Here's how the part is built. I have some questions about the finished solid (model axes, mm). Face numbers are marked on the shaded views. A direction names the side the tool comes from. Give positions to 0.01 mm unless a question says otherwise; leave off trailing zeros. Loops run counter-clockwise (first coordinate to the right, second up) from the corner with the lowest first, then second, coordinate; pieces in that order, holes last. Notation, with made-up numbers: (-11.75, 37) - (29.25, 37) arc R9 cw to (29.25, 50) - close; hole circle Ø6 at (54.5, 31). An arc over 180 degrees is marked (long way). One line per item, written item: value. Start each with the question number.
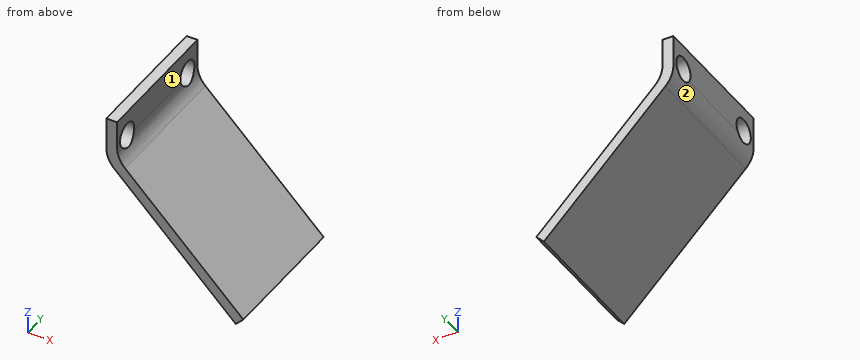
```python
from build123d import *

# Parameters (mm, degrees)
SKETCH1_W               = 1
SKETCH1_H               = 4
BOSS_EXTRUDE1_DEPTH     = 12.7
BOSS_EXTRUDE2_DEPTH     = 12.7
FILLET1_R               = 2.54
SKETCH3_R               = 1.125
CUT_EXTRUDE1_DEPTH      = 24.536198366
CUT_EXTRUDE1_DEPTH_BACK = 24.536198366


with BuildPart() as part:
    # Sketch1 → Boss-Extrude1 (new body)
    with BuildSketch(Plane(origin=(0, 0, 0), x_dir=(1, 0, 0), z_dir=(0, 1, 0))):
        with Locations((0.5, 2)):
            Rectangle(SKETCH1_W, SKETCH1_H)
    extrude(amount=BOSS_EXTRUDE1_DEPTH)

    # Sketch2 → Boss-Extrude2 (add)
    with BuildSketch(Plane(origin=(0, 0, 0), x_dir=(1, 0, 0), z_dir=(0, 1, 0))):
        Polygon((0, 4), (11.992893219, 15.992893219), (12.7, 15.285786438), (0.707106781, 3.292893219), align=None)
    extrude(amount=BOSS_EXTRUDE2_DEPTH)

    # Fillet1
    fillet1_edges = [part.edges().sort_by_distance(p)[0] for p in [
        (1, 6.35, -3.585786438),
        (0, 6.35, -4),
    ]]
    fillet(fillet1_edges, radius=FILLET1_R)

    # Sketch3 → Cut-Extrude1 (cut, two sides)
    with BuildSketch(Plane(origin=(1, 0, 0), x_dir=(0, 0, -1), z_dir=(1, 0, 0))) as cut_extrude1_sk:
        with Locations(Location((2.276792488, 11.1125, 0), (0, 0, 306.622338606))):
            Circle(SKETCH3_R)
        with Locations(Location((2.276792488, 1.5875, 0), (0, 0, 306.622338606))):
            Circle(SKETCH3_R)
    extrude(amount=CUT_EXTRUDE1_DEPTH, mode=Mode.SUBTRACT)
    extrude(cut_extrude1_sk.sketch, amount=-CUT_EXTRUDE1_DEPTH_BACK, mode=Mode.SUBTRACT)


solid = part.part
```
(1) If we section it at D-D on x = 3.5: List the corners of the cut face in (y, z) for me.
(2) If we section it at B-B on y = 6.5: List the corners of the cut face in (x, z) for me.
(3) Will these pins go through, and if not, where does the flat tip stop? pin 1 (1.5 mm diameter, centred on x = 3, y = 6, fed in from +Z); pin 2 (6 mm diameter, centred on y = 10, z = -12.5, fed in from -X); pin 3 (3 mm diameter, centred on y = 8, z = -1.5, fed in from +X); pin 4 (2 mm diameter, centred on x = 5.5, z = -7, fed in from -Y).
(4) For the marked faces 1 and 2, which set-ups out of +Z, -Z, +X, -X, +Y, -Y let a thin tool reach every point of the face, with its end or its side?
(5) If we section it at A-A on y = 11: List the corners of the cut face in (x, z) for me, plus the area to 3 significant figures.
(6) If we section it at C-C on z = -13: List the corners of the cut face in (x, y) for me.
(7) Please list where these lines run through material, in increasing order: probe 1 along X at (y, z) = (9.25, -2); probe 2 along Z at (x, y) = (5.75, 4.75); probe 3 along X at (y, z) = (6, -9.5). Write a range as from..to.
Found:
1. outline: (0, -7.5) - (12.7, -7.5) - (12.7, -6.09) - (0, -6.09) - close
2. outline: (0, -2.95) arc R2.54 ccw to (0.74, -4.74) - (11.99, -15.99) - (12.7, -15.29) - (1.74, -4.33) arc R2.54 cw to (1, -2.53) - (1, 0) - (0, 0) - close
3. pin 1: z = -4.84
3. pin 2: x = 5.5
3. pin 3: x = 1.04
3. pin 4: y = 0
4. face 1: +Z, +X, +Y, -Y
4. face 2: -Z, -X, +Y, -Y
5. outline: (0, -1.16) - (1, -1.16) - (1, 0) - (0, 0) - close; (0.04, -3.4) arc R2.54 ccw to (0.74, -4.74) - (11.99, -15.99) - (12.7, -15.29) - (1.74, -4.33) arc R2.54 cw to (1.15, -3.4) - close
5. area: 18.3 mm^2
6. outline: (9, 0) - (10.41, 0) - (10.41, 12.7) - (9, 12.7) - close
7. probe 1: 0..1
7. probe 2: -9.75..-8.34
7. probe 3: 5.5..6.91
